from build123d import *

# Parameters (mm, degrees)
SKETCH2_W           = 125
SKETCH2_H           = 125
SKETCH2_R           = 1.5
SKETCH2_R_2         = 2.5
BOSS_EXTRUDE1_DEPTH = 10.5
CUT_EXTRUDE1_DEPTH  = 5


with BuildPart() as part:
    # Sketch2 → Boss-Extrude1 (new body)
    with BuildSketch(Plane.XY):
        with Locations((29.251653193, -12.17)):
            Rectangle(SKETCH2_W, SKETCH2_H)
        with Locations((-25.5, -2)):
            Circle(SKETCH2_R, mode=Mode.SUBTRACT)
        with Locations((25.5, -2)):
            Circle(SKETCH2_R, mode=Mode.SUBTRACT)
        with Locations((78.251653193, 0.33)):
            Circle(SKETCH2_R_2, mode=Mode.SUBTRACT)
        with Locations((36.251653193, 0.33)):
            Circle(SKETCH2_R_2, mode=Mode.SUBTRACT)
        with Locations((36.251653193, -67.67)):
            Circle(SKETCH2_R_2, mode=Mode.SUBTRACT)
        with Locations((78.251653193, -67.67)):
            Circle(SKETCH2_R_2, mode=Mode.SUBTRACT)
        with Locations((25.5, 44.5)):
            Circle(SKETCH2_R, mode=Mode.SUBTRACT)
        with Locations((-25.5, 44.5)):
            Circle(SKETCH2_R, mode=Mode.SUBTRACT)
    extrude(amount=BOSS_EXTRUDE1_DEPTH)

    # Sketch3 → Cut-Extrude1 (cut)
    with BuildSketch(Plane.XY.offset(10.5)):
        Polygon((74.316653193, -69.941873309), (78.251653193, -72.213746619), (82.186653193, -69.941873309), (82.186653193, -65.398126691), (78.251653193, -63.126253381), (74.316653193, -65.398126691), align=None)
        Polygon((36.251653193, -72.213746619), (40.186653193, -69.941873309), (40.186653193, -65.398126691), (36.251653193, -63.126253381), (32.316653193, -65.398126691), (32.316653193, -69.941873309), align=None)
        Polygon((36.251653193, -4.213746619), (40.186653193, -1.941873309), (40.186653193, 2.601873309), (36.251653193, 4.873746619), (32.316653193, 2.601873309), (32.316653193, -1.941873309), align=None)
        Polygon((78.251653193, -4.213746619), (82.186653193, -1.941873309), (82.186653193, 2.601873309), (78.251653193, 4.873746619), (74.316653193, 2.601873309), (74.316653193, -1.941873309), align=None)
        Polygon((22.785, -3.567505981), (25.5, -5.135011962), (28.215, -3.567505981), (28.215, -0.432494019), (25.5, 1.135011962), (22.785, -0.432494019), align=None)
        Polygon((-28.215, -3.567505981), (-25.5, -5.135011962), (-22.785, -3.567505981), (-22.785, -0.432494019), (-25.5, 1.135011962), (-28.215, -0.432494019), align=None)
        Polygon((22.785, 42.932494019), (25.5, 41.364988038), (28.215, 42.932494019), (28.215, 46.067505981), (25.5, 47.635011962), (22.785, 46.067505981), align=None)
        Polygon((-28.215, 42.932494019), (-25.5, 41.364988038), (-22.785, 42.932494019), (-22.785, 46.067505981), (-25.5, 47.635011962), (-28.215, 46.067505981), align=None)
    extrude(amount=-CUT_EXTRUDE1_DEPTH, mode=Mode.SUBTRACT)


solid = part.part
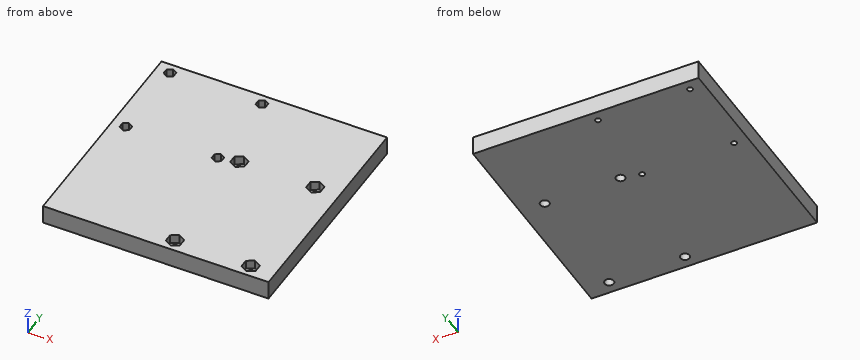
Input: part model. Units: mm. Frame: model coordinates. Give positions to 0.01 mm unless a question says otherwise; leave off trailing zeros. Write each loop counter-clockwise with the first axis right and the second up, starting at its lowest first coordinate (ties: lowest second). Pieces come first, ordered by that corner, then holes.
Q1. Section C-C, the plane z = 8.25. State how many separate pieces and enclosed holes the cut face has, plus the area to 3 significant figures.
Q2. Section B-B, the plane y = -67.67. Output: boundary loops of the cut face in (x, z).
Q3. Section A-A, the plane y = 44.5. Output: boundary loops of the cut face in (x, z) (3 decimals), plus the area to 3 significant figures.
Q4. First-contact query: P1, Ø6, axis at x = -26, y = 45, coming from the +Z side; P2, Ø3, axis at x = 78.25, y = 0.33, coming from the -Z side; P3, Ø3.5, axis at x = -25.5, y = 44.5, coming from the +Z side. Flat tips, straight axial feed; report the tip coordinate or a pass-through.
Q5. Material intervals for probe 1 along X at (y, z) = (44.5, 1.65); probe 2 along X at (y, z) = (-67.67, 2.65); probe 3 along Y at (x, z) = (-25.5, 1.15), sorted ascending.
Filled in:
1. separate pieces: 1
1. enclosed holes: 8
1. area: 15,300 mm2
2. outline: (-33.25, 0) - (33.75, 0) - (33.75, 5.5) - (32.32, 5.5) - (32.32, 10.5) - (-33.25, 10.5) - close; (38.75, 0) - (75.75, 0) - (75.75, 5.5) - (74.32, 5.5) - (74.32, 10.5) - (40.19, 10.5) - (40.19, 5.5) - (38.75, 5.5) - close; (80.75, 0) - (91.75, 0) - (91.75, 10.5) - (82.19, 10.5) - (82.19, 5.5) - (80.75, 5.5) - close
3. outline: (-33.248, 0) - (-27, 0) - (-27, 5.5) - (-28.215, 5.5) - (-28.215, 10.5) - (-33.248, 10.5) - close; (-24, 0) - (24, 0) - (24, 5.5) - (22.785, 5.5) - (22.785, 10.5) - (-22.785, 10.5) - (-22.785, 5.5) - (-24, 5.5) - close; (27, 0) - (91.752, 0) - (91.752, 10.5) - (28.215, 10.5) - (28.215, 5.5) - (27, 5.5) - close
3. area: 1,230 mm2
4. P1: stops at z = 10.5
4. P2: passes through
4. P3: stops at z = 5.5
5. probe 1: x = -33.25 to -27, -24 to 24, 27 to 91.75
5. probe 2: x = -33.25 to 33.75, 38.75 to 75.75, 80.75 to 91.75
5. probe 3: y = -74.67 to -3.5, -0.5 to 43, 46 to 50.33
